The drawing under review shows one solid part. Ordinate dimensions are in mm from its lowest x, y, z. A direction names the side the tool comes from. Give positions to 0.01 mm unless a question says otherwise; leave off trailing zeros. Write each loop counter-clockwise with the first axis right and the second up, starting at its lowest first coordinate (ties: lowest second). Pieces come first, ordered by that corner, then holes. Notation, with made-up numbers: (24, 68) -> (67, 68) arc R10 ccw to (67, 75) -> close; hole circle Ø8 at (87.25, 40). An arc over 180 degrees is marked (long way). Answer as a JSON object with one key per item and string values.
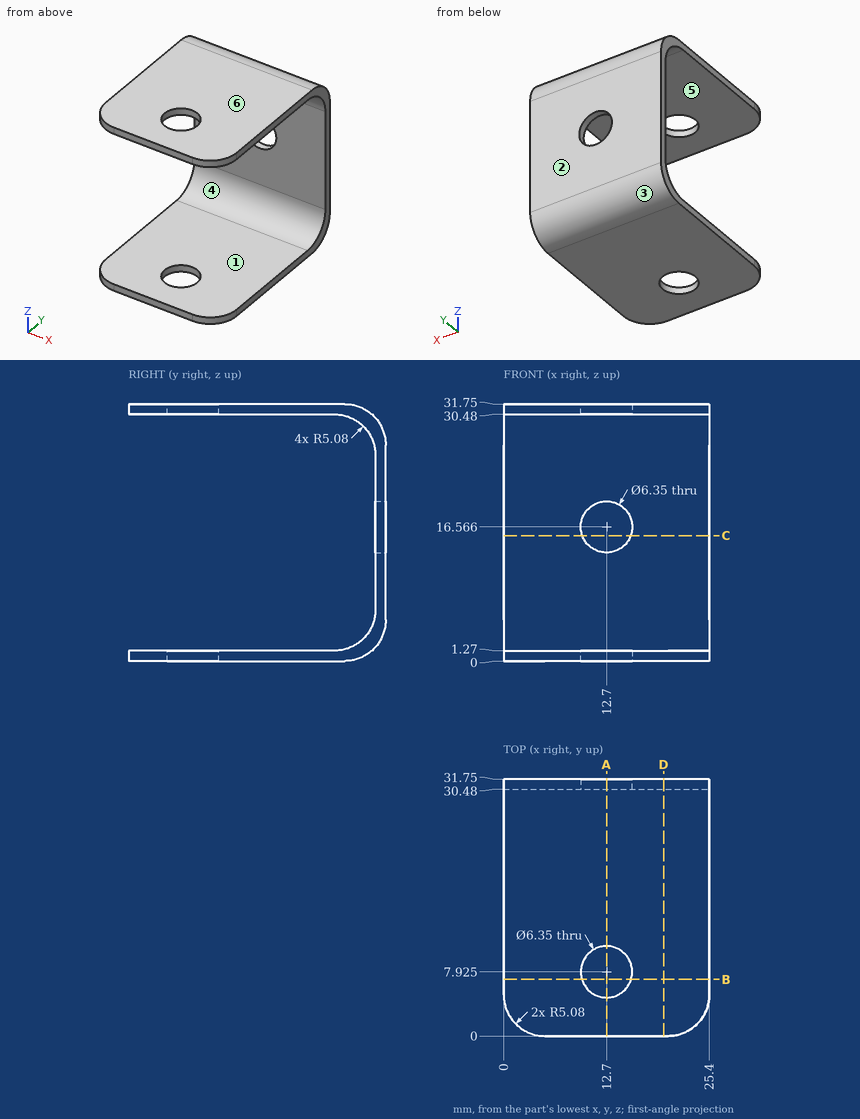
(1) We need section B-B, the plane y = 7. State the section outline as (x, z) points.
Here are the results:
{"outline": "(0, 0) -> (9.66, 0) -> (9.66, 1.27) -> (0, 1.27) -> close; (0, 30.48) -> (9.66, 30.48) -> (9.66, 31.75) -> (0, 31.75) -> close; (15.74, 0) -> (25.4, 0) -> (25.4, 1.27) -> (15.74, 1.27) -> close; (15.74, 30.48) -> (25.4, 30.48) -> (25.4, 31.75) -> (15.74, 31.75) -> close"}
(2) For the marked faces 5 and 6, list the 3-axis set-ups (+Z, -Z, +X, -X, +Y, -Y) from which the entire face can be reached by the end or side of a thin tool; tool diameter is ignored.
Here are the results:
{"face 5": "+X, -X, -Y", "face 6": "+Z, +X, -X, +Y, -Y"}
(3) The part is to be moulded in two halves that separate along Z. For the marked faces 1, 2, 3 and 4, say which applies: +Z half, -Z half, draft (parallel to the pull), parting line (faces both ways), or undercut.
Here are the results:
{"face 1": "undercut", "face 2": "draft", "face 3": "-Z half", "face 4": "undercut"}
(4) For line 1 along Z through (x, y) = (21.5, 5); line 2 along Y through (x, z) = (20.5, 23); line 3 along Y through (x, z) = (12.7, 31.25), list the stretches that pass through material, from the lowest coordinate up.
Here are the results:
{"line 1": "z = 0 to 1.27, 30.48 to 31.75", "line 2": "y = 30.48 to 31.75", "line 3": "y = 0 to 4.75, 11.1 to 28.87"}
(5) We need section C-C, the plane z = 15.5. State the section outline as (x, y) points.
Here are the results:
{"outline": "(0, 30.48) -> (9.71, 30.48) -> (9.71, 31.75) -> (0, 31.75) -> close; (15.69, 30.48) -> (25.4, 30.48) -> (25.4, 31.75) -> (15.69, 31.75) -> close"}
(6) We need section A-A, the plane x = 12.7. State the section outline as (y, z) points.
Here are the results:
{"outline": "(0, 0) -> (4.75, 0) -> (4.75, 1.27) -> (0, 1.27) -> close; (0, 30.48) -> (4.75, 30.48) -> (4.75, 31.75) -> (0, 31.75) -> close; (11.1, 0) -> (26.67, 0) arc R5.08 ccw to (31.75, 5.08) -> (31.75, 13.39) -> (30.48, 13.39) -> (30.48, 6.35) arc R5.08 cw to (25.4, 1.27) -> (11.1, 1.27) -> close; (11.1, 30.48) -> (25.4, 30.48) arc R5.08 cw to (30.48, 25.4) -> (30.48, 19.74) -> (31.75, 19.74) -> (31.75, 26.67) arc R5.08 ccw to (26.67, 31.75) -> (11.1, 31.75) -> close"}
(7) Clearance check with flat-ended pins moving along their axes: pin 1 (5.5 mm diameter, centred on x = 14.5, z = 17, fed in from -Y); pin 2 (5 mm diameter, centred on x = 12.7, y = 7.92, fed in from -Z). State where each tip first meets the part, or that it passes through.
Here are the results:
{"pin 1": "stops at y = 30.48", "pin 2": "passes through"}
(8) We need section D-D, the plane x = 19.75. State the section outline as (y, z) points.
Here are the results:
{"outline": "(0, 0) -> (26.67, 0) arc R5.08 ccw to (31.75, 5.08) -> (31.75, 26.67) arc R5.08 ccw to (26.67, 31.75) -> (0, 31.75) -> (0, 30.48) -> (25.4, 30.48) arc R5.08 cw to (30.48, 25.4) -> (30.48, 6.35) arc R5.08 cw to (25.4, 1.27) -> (0, 1.27) -> close"}
